For this review, take the finished solid that the model builds, in its own axes (mm). Give positions to 0.01 mm unless a question says otherwise; leave off trailing zeros. Write each loop counter-clockwise with the first axis right and the second up, starting at its lowest first coordinate (ties: lowest second). Pieces come first, ordered by that corner, then holes.
from build123d import *

# Parameters (mm, degrees)
F1_DEPTH = 6
F2_SIZE  = 5.99999
F3_W     = 4.9
F3_H     = 9
F3_R     = 1.5
F4_DEPTH = 6


# Not quite as in the source:
# - a fillet or chamfer is up to 0.001 mm smaller than in the source, because OpenCascade refuses the exact size


with BuildPart() as f1:
    # F0 (on Top) → F1 (new body)
    with BuildSketch(Plane.XY):
        Polygon((-367.6438903809, 71.5354757011), (-372.5438903809, 71.5354757011), (-372.5438903809, 44.0354757011), (-367.6438903809, 41.5354757011), align=None)
    extrude(amount=F1_DEPTH)

    # F2 (size 6 in the source; OpenCascade refuses exactly that, so slightly less here)
    f2_edges = [f1.edges().sort_by_distance(p)[0] for p in [
        (-370.09389, 42.785476, 0),
    ]]
    chamfer(f2_edges, length=F2_SIZE)

    # F3 (on face) → F4 (cut, through all)
    with BuildSketch(Plane.XY.offset(6)):
        with Locations((-370.0938903809, 67.0354757011)):
            Rectangle(F3_W, F3_H)
        with Locations((-370.0938903809, 59.0354757011)):
            Circle(F3_R)
        with Locations((-370.0938903809, 54.0354757011)):
            Circle(F3_R)
    extrude(amount=-F4_DEPTH, mode=Mode.SUBTRACT)


solid = f1.part
(1) We need section B-B (z = 3.2). Write out the cut boundary in (x, y).
(2) The part is to be moulded in two halves that separate along Y. For faces 1 (the flat face through (-370.128, 46.218, 2.958)), 2 (the cylindrical face through (-368.663, 54.486, 3.042)), 3 (the flat face through (-370, 62.535, 3)), say which applies: +Y half, -Y half, draft (parallel to the pull), parting line (faces both ways), or undercut.
(3) We need section C-C (y = 53.5). Write out the cut boundary in (x, z), and give its area (3 significant figures).
(4) We need section A-A (x = -370.6). Count the separate pieces of the cut face and the enclosed holes in it, and give its area (3 significant figures).
(5) For L1, parallel to Y at x = -369.45, z = 3.3; L2, parallel to Y at x = -371.15, z = 4.75; L3, parallel to X at y = 55, z = 5.05, list the stretches that pass through material, from the lowest coordinate up.
The answers:
1. outline: (-372.54, 47.18) - (-367.64, 44.68) - (-367.64, 62.54) - (-372.54, 62.54) - close; hole circle Ø3 at (-370.09, 54.04); hole circle Ø3 at (-370.09, 59.04)
2. face 1: -Y half
2. face 2: undercut
2. face 3: +Y half
3. outline: (-372.54, 0) - (-371.5, 0) - (-371.5, 6) - (-372.54, 6) - close; (-368.69, 0) - (-367.64, 0) - (-367.64, 6) - (-368.69, 6) - close
3. area: 12.6 mm2
4. separate pieces: 3
4. enclosed holes: 0
4. area: 62.9 mm2
5. L1: y = 45.49 to 52.68, 55.39 to 57.68, 60.39 to 62.54
5. L2: y = 44.73 to 52.97, 55.1 to 57.97, 60.1 to 62.54
5. L3: x = -372.54 to -371.24, -368.95 to -367.64
